Can you work these out from the model? Positions are in its coordinate system, mm. Face numbers are marked on the shaded views. A direction names the side the tool comes from. Coordinates: 2 decimals unless noted, no trailing zeros. Write each loop counter-clockwise with the first axis right and the second up, starting at its lowest first coordinate (ties: lowest second). Pieces come first, ordered by that corner, then holes. Notation, with made-up numbers: (-19, 46) - (22, 46) arc R8 cw to (22, 59) - close; hole circle Ø9 at (-11.5, -34). An arc over 180 degrees is marked (long way). One line per question, with ' | ' between items. Start each with the question number.
from build123d import *

# Parameters (mm, degrees)
SKETCH_1_W          = 80
SKETCH_1_H          = 35
EXTRUDE_1_DEPTH     = 2
SKETCH_2_W          = 80
SKETCH_2_H          = 35
SKETCH_2_W_2        = 76
SKETCH_2_H_2        = 31
EXTRUDE_2_DEPTH     = 16
SKETCH_3_W          = 10.5
SKETCH_3_H          = 12.5
CUT_EXTRUDE_1_DEPTH = 81
SKETCH_4_R          = 1.15
SKETCH_4_R_2        = 1.75
CUT_EXTRUDE_2_DEPTH = 3
CUT_EXTRUDE_3_DEPTH = 19
CUT_EXTRUDE_4_REACH = 37
SKETCH_6_W          = 12.7
SKETCH_6_H          = 3
CUT_EXTRUDE_5_REACH = 37
SKETCH_7_W          = 12.7
SKETCH_7_H          = 11.63


with BuildPart() as part:
    # 草图1 → 凸台-拉伸1 (new body)
    with BuildSketch(Plane.XY):
        Rectangle(SKETCH_1_W, SKETCH_1_H)
    extrude(amount=EXTRUDE_1_DEPTH)

    # 草图2 → 凸台-拉伸2 (add)
    with BuildSketch(Plane.XY.offset(2)):
        Rectangle(SKETCH_2_W, SKETCH_2_H)
        Rectangle(SKETCH_2_W_2, SKETCH_2_H_2, mode=Mode.SUBTRACT)
    extrude(amount=EXTRUDE_2_DEPTH)

    # 草图3 → 切除-拉伸1 (cut, through all)
    with BuildSketch(Plane.ZY.offset(40)):
        with Locations((8.85, 0)):
            Rectangle(SKETCH_3_W, SKETCH_3_H)
    extrude(amount=-CUT_EXTRUDE_1_DEPTH, mode=Mode.SUBTRACT)

    # 草图4 → 切除-拉伸2 (cut, through all)
    with BuildSketch(Plane.XY.offset(2)):
        with Locations((-29.5, 9.140333749)):
            Circle(SKETCH_4_R)
        with Locations((-29.5, -8.859666251)):
            Circle(SKETCH_4_R)
        with Locations((29.5, 9.140333749)):
            Circle(SKETCH_4_R)
        with Locations((29.5, -8.859666251)):
            Circle(SKETCH_4_R)
        with Locations((-15, 0)):
            Circle(SKETCH_4_R_2)
        with Locations((15, 0)):
            Circle(SKETCH_4_R_2)
    extrude(amount=-CUT_EXTRUDE_2_DEPTH, mode=Mode.SUBTRACT)

    # 草图5 → 切除-拉伸3 (cut, through all)
    with BuildSketch(Plane(origin=(0, 0, 0), x_dir=(-1, 0, 0), z_dir=(0, 0, -1))):
        with BuildLine():
            Line((-8.89, 13.468), (8.89, 13.468))
            ThreePointArc((8.89, 13.468), (10.16, 12.198), (8.89, 10.928))
            Line((8.89, 10.928), (-8.89, 10.928))
            ThreePointArc((-8.89, 10.928), (-10.16, 12.198), (-8.89, 13.468))
        make_face()
        with BuildLine():
            Line((-8.89, -1.772), (8.89, -1.772))
            ThreePointArc((8.89, -1.772), (10.16, -3.042), (8.89, -4.312))
            Line((8.89, -4.312), (-8.89, -4.312))
            ThreePointArc((-8.89, -4.312), (-10.16, -3.042), (-8.89, -1.772))
        make_face()
        with BuildLine():
            Line((-22.098, 12.706), (-11.938, 12.706))
            ThreePointArc((-11.938, 12.706), (-10.668, 11.436), (-11.938, 10.166))
            Line((-11.938, 10.166), (-22.098, 10.166))
            ThreePointArc((-22.098, 10.166), (-23.368, 11.436), (-22.098, 12.706))
        make_face()
        with BuildLine():
            Line((11.94, 12.706), (22.1, 12.706))
            ThreePointArc((22.1, 12.706), (23.37, 11.436), (22.1, 10.166))
            Line((22.1, 10.166), (11.94, 10.166))
            ThreePointArc((11.94, 10.166), (10.67, 11.436), (11.94, 12.706))
        make_face()
    extrude(amount=-CUT_EXTRUDE_3_DEPTH, mode=Mode.SUBTRACT)

    # 草图6 → 切除-拉伸4 (cut, up to next)
    with BuildSketch(Plane(origin=(0, 17.5, 0), x_dir=(1, 0, 0), z_dir=(0, 1, 0)), mode=Mode.PRIVATE) as cut_extrude_4_sk1:
        with Locations((-17.018, -4.87)):
            Rectangle(SKETCH_6_W, SKETCH_6_H)
    cut_extrude_4_tool1 = extrude(cut_extrude_4_sk1.sketch, amount=-CUT_EXTRUDE_4_REACH, mode=Mode.PRIVATE) & part.part
    add(cut_extrude_4_tool1.solids().sort_by_distance((-17.018, 17.5, 4.87))[0], mode=Mode.SUBTRACT)
    # 草图6 → 切除-拉伸4 (cut, up to next)
    with BuildSketch(Plane(origin=(0, 17.5, 0), x_dir=(1, 0, 0), z_dir=(0, 1, 0)), mode=Mode.PRIVATE) as cut_extrude_4_sk2:
        with Locations((17.02, -4.87)):
            Rectangle(SKETCH_6_W, SKETCH_6_H)
    cut_extrude_4_tool2 = extrude(cut_extrude_4_sk2.sketch, amount=-CUT_EXTRUDE_4_REACH, mode=Mode.PRIVATE) & part.part
    add(cut_extrude_4_tool2.solids().sort_by_distance((17.02, 17.5, 4.87))[0], mode=Mode.SUBTRACT)

    # 草图7 → 切除-拉伸5 (cut, up to next)
    with BuildSketch(Plane(origin=(0, 17.5, 0), x_dir=(1, 0, 0), z_dir=(0, 1, 0)), mode=Mode.PRIVATE) as cut_extrude_5_sk1:
        with Locations((-17.018, -12.185)):
            Rectangle(SKETCH_7_W, SKETCH_7_H)
    cut_extrude_5_tool1 = extrude(cut_extrude_5_sk1.sketch, amount=-CUT_EXTRUDE_5_REACH, mode=Mode.PRIVATE) & part.part
    add(cut_extrude_5_tool1.solids().sort_by_distance((-17.018, 17.5, 12.185))[0], mode=Mode.SUBTRACT)
    # 草图7 → 切除-拉伸5 (cut, up to next)
    with BuildSketch(Plane(origin=(0, 17.5, 0), x_dir=(1, 0, 0), z_dir=(0, 1, 0)), mode=Mode.PRIVATE) as cut_extrude_5_sk2:
        with Locations((17.02, -12.185)):
            Rectangle(SKETCH_7_W, SKETCH_7_H)
    cut_extrude_5_tool2 = extrude(cut_extrude_5_sk2.sketch, amount=-CUT_EXTRUDE_5_REACH, mode=Mode.PRIVATE) & part.part
    add(cut_extrude_5_tool2.solids().sort_by_distance((17.02, 17.5, 12.185))[0], mode=Mode.SUBTRACT)


solid = part.part
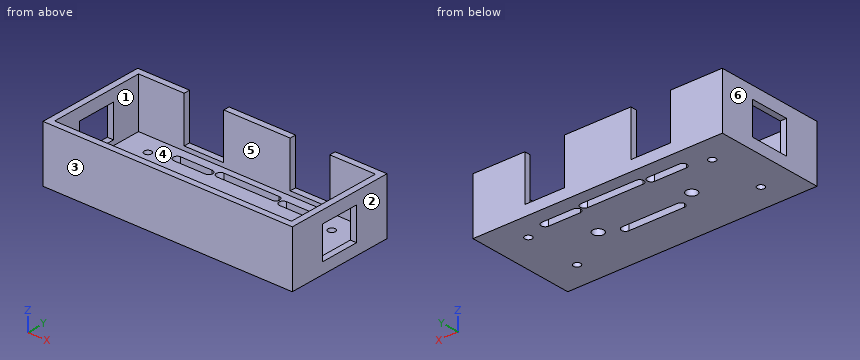
(1) If we section it at D-D on x = -8: List the corners of the cut face in (y, z) for me.
(2) Which directions (+Z, -Z, +X, -X, +Y, -Y) give clear straight access to the entire face, cutting with the end or side of a thin tool? Please do the marked faces 1 and 2.
(3) I'm going to push flat-ended pins straight in: pin 1 (4 mm diameter, centred on x = -18, y = -3, fed in from +Z); pin 2 (3 mm diameter, centred on x = -15, y = 0, fed in from +Z); pin 3 (2 mm diameter, centred on x = -16, y = 16, fed in from +Z). Where does each tip first touch, or does it pass through?
(4) If we section it at B-B on y = 0: List the corners of the cut face in (x, z) for me.
(5) If we section it at C-C on z = 5: List the corners of the cut face in (x, y) for me.
(6) If we mould it in two halves opening along Y, with no side actions, what happens to the marked faces 3, 4, 5 and 6? For each: +Y half, -Y half, draft (parallel to the pull), parting line (faces both ways), or undercut.
(7) If we section it at A-A on x = 15: List the corners of the cut face in (y, z) for me, plus the area to 3 significant figures.
(8) If I drill on probe 1 along Y at (x, z) = (-29.5, 0.95); probe 2 along Y at (x, z) = (15, 1); probe 3 along X at (y, z) = (3.5, 17.25), over which ranges is the centre line in solid material (lowest first)?
Values:
1) outline: (-17.5, 0) - (-4.31, 0) - (-4.31, 2) - (-15.5, 2) - (-15.5, 18) - (-17.5, 18) - close; (-1.77, 0) - (10.93, 0) - (10.93, 2) - (-1.77, 2) - close; (13.47, 0) - (17.5, 0) - (17.5, 18) - (15.5, 18) - (15.5, 2) - (13.47, 2) - close
2) face 1: +Z | face 2: +Z, -Z, +X, +Y, -Y
3) pin 1: z = 2 | pin 2: through | pin 3: z = 3.37
4) outline: (-40, 0) - (-16.75, 0) - (-16.75, 2) - (-38, 2) - (-38, 3.6) - (-40, 3.6) - close; (-40, 14.1) - (-38, 14.1) - (-38, 18) - (-40, 18) - close; (-13.25, 0) - (13.25, 0) - (13.25, 2) - (-13.25, 2) - close; (16.75, 0) - (40, 0) - (40, 3.6) - (38, 3.6) - (38, 2) - (16.75, 2) - close; (38, 14.1) - (40, 14.1) - (40, 18) - (38, 18) - close
5) outline: (-40, -17.5) - (40, -17.5) - (40, -6.25) - (38, -6.25) - (38, -15.5) - (-38, -15.5) - (-38, -6.25) - (-40, -6.25) - close; (-40, 6.25) - (-38, 6.25) - (-38, 15.5) - (-23.37, 15.5) - (-23.37, 17.5) - (-40, 17.5) - close; (-10.67, 15.5) - (10.67, 15.5) - (10.67, 17.5) - (-10.67, 17.5) - close; (23.37, 15.5) - (38, 15.5) - (38, 6.25) - (40, 6.25) - (40, 17.5) - (23.37, 17.5) - close
6) face 3: -Y half | face 4: undercut | face 5: undercut | face 6: draft
7) outline: (-17.5, 0) - (-1.75, 0) - (-1.75, 2) - (-15.5, 2) - (-15.5, 18) - (-17.5, 18) - close; (1.75, 0) - (10.17, 0) - (10.17, 2) - (1.75, 2) - close; (12.71, 0) - (17.5, 0) - (17.5, 3.37) - (15.5, 3.37) - (15.5, 2) - (12.71, 2) - close | area: 92.7 mm2
8) probe 1: -17.5 to -10.01, -7.71 to 7.99, 10.29 to 17.5 | probe 2: -17.5 to -1.75, 1.75 to 10.17, 12.71 to 17.5 | probe 3: -40 to -38, 38 to 40
